Autodesk Inventor part; units mm, degrees
ref_plane "YZ Plane" through (0, 0, 0) normal (1, 0, 0) x (0, 1, 0)
ref_plane "XZ Plane" through (0, 0, 0) normal (0, 1, 0) x (-1, 0, 0)
ref_plane "XY Plane" through (0, 0, 0) normal (0, 0, 1) x (1, 0, 0)
sketch "Sketch1" plane through (0, 0, 0) normal (0, 1, 0) x (-1, 0, 0)
  circle A0 centre (0, 0) radius 19.05
  dimension "d0" = 38.1
extrude "Extrusion1" add sketch "Sketch1" along normal blind 2.794
hole "Hole1" at (0, 2.794, 0) direction (0, -1, 0) diameter 21.082 end through all
chamfer "Chamfer1" distance 1.397 angle 45 1 edges at (0, 0, -10.541)
properties part number "Switch Hole Test"
Verification items for the finished model (mm, model axes). Coordinates: 2 decimals unless noted, no trailing zeros. Order: outer loops, then holes, each group sorted by start corner. A loop starts at its lowest first (then second) coordinate and runs counter-clockwise, first axis right, second up. Notation, with made-up numbers: M 82.5,83.5 L 97.5,83.5 A19 ccw 97.5,95.5 Z; hole C 21.25,-2 d10. An arc over 180 degrees is marked long. One line per item, written item: value. Start each with the question number.
Item 1: Sectioned sample at A-A (z = 0). Enter the section's corners in (x, y), then the cut area to 3 significant figures.
Item 2: Scan lines: probe 1 along Z at (x, y) = (0, 2.4); probe 2 along Z at (x, y) = (-3.5, 0.55); probe 3 along X at (y, z) = (2.05, 3). Record each from-to range of solid material in increasing order.
Item 3: Sectioned sample at C-C (y = 0.5). Enter the section's corners in (x, z).
Item 4: Sectioned sample at B-B (x = 0). Enter the section's corners in (y, z), then the cut area to 3 significant figures.
Item 5: Mould release check, pull along Z, two halves, no side actions. Record for faces 1 (the cylindrical face through (-3.166, 2.086, 10.054)), 2 (the flat face through (-8, 2.794, -8)), 3 (the cylindrical face through (15.12, 1.38, 11.59)): released by +Z, released by -Z, zero draft, split by the parting line, or undercut.
Conclusion:
1. outline: M -19.05,0 L -11.94,0 L -10.54,1.4 L -10.54,2.79 L -19.05,2.79 Z; M 10.54,1.4 L 11.94,0 L 19.05,0 L 19.05,2.79 L 10.54,2.79 Z
1. area: 45.6 mm^2
2. probe 1: z = -19.05 to -10.54, 10.54 to 19.05
2. probe 2: z = -18.73 to -10.84, 10.84 to 18.73
2. probe 3: x = -18.81 to -10.11, 10.11 to 18.81
3. outline: C 0,0 d38.1; hole C 0,0 d22.88
4. outline: M 0,-19.05 L 2.79,-19.05 L 2.79,-10.54 L 1.4,-10.54 L 0,-11.94 Z; M 0,11.94 L 1.4,10.54 L 2.79,10.54 L 2.79,19.05 L 0,19.05 Z
4. area: 45.6 mm^2
5. face 1: undercut
5. face 2: zero draft
5. face 3: split by the parting line
